The model under review builds one solid part; all positions refer to its coordinate system, in mm. A direction names the side the tool comes from. Coordinates: 2 decimals unless noted, no trailing zeros. Order: outer loops, then holes, each group sorted by start corner. A loop starts at its lowest first (then second) coordinate and runs counter-clockwise, first axis right, second up. Notation, with made-up numbers: (-13, 15.5) -> (29, 15.5) arc R17 ccw to (29, 29.5) -> close; hole circle Ø10 at (80.25, -26). An arc over 180 degrees is marked (long way). Use one line per item in the form item = value. Start each with the question number.
(1) Wall thickness on line 1 along X through (y, z) = (304.45, 5.5); line 2 along Y through (x, z) = (-935.75, 6.25); line 3 along X through (y, z) = (304.2, -3): over which ranges is each line inside the solid? List them lowest first.
(2) Take a section at C-C (x = -935). State the section outline as (y, z) points.
(3) Take a section at B-B (x = -944.25). State the section outline as (y, z) points.
(4) Take a section at D-D (y = 302.3). State the section outline as (x, z) points.
(5) Take a section at A-A (z = -7.5). State the section outline as (x, y) points.
(6) Mouldability with a two-part tool opening along X and no side actions: class faces 1 (the cylindrical face through (-942.71, 304.69, -0.13)), 2 (the cylindrical face through (-943.634, 306.887, -0.133)), 3 (the cylindrical face through (-946.211, 303.218, -0.133)), 4 (the flat face through (-934, 304, -9.5)) as +X half, -X half, draft (parallel to the pull), parting line (faces both ways), or undercut.
(7) For faces 5 (the flat face through (-930, 305.387, 0)), 6 (the flat face through (-948, 303.387, 0)), 7 (the flat face through (-930, 303.387, 0)), 8 (the flat face through (-948, 305.387, 0)), list the 3-axis set-ups (+Z, -Z, +X, -X, +Y, -Y) from which the entire face can be reached by the end or side of a thin tool; tool diameter is ignored.
(8) Insertion check: pin 1 Ø0.5 at (x, z) = (-947.5, -3.5) entering from -Y; pin 2 Ø4 at (x, z) = (-924, 6.5) entering from +Y; pin 3 Ø2 at (y, z) = (306, 0) entering from +X; pin 4 Ø1.6 at (x, y) = (-943.66, 304.39) entering from +Z. Each pin has a flat end and moves straight along its axis. Give the tip position at first contact, or say it passes through.
```python
from build123d import *

# Parameters (mm, degrees)
BOSS_EXTRUDE1_DEPTH      = 9.5
BOSS_EXTRUDE1_DEPTH_BACK = 9.5
SKETCH1_R                = 1


with BuildPart() as part:
    # Sketch1 → Boss-Extrude1 (new, two sides: drawn at the far end of the back side and taken through both)
    with BuildSketch(Plane.XY.offset(-BOSS_EXTRUDE1_DEPTH_BACK)):
        with BuildLine():
            Line((-948.662974387, 303.387338025), (-947.017076353, 303.387338025))
            ThreePointArc((-947.017076353, 303.387338025), (-946.200579773, 303.213079884), (-945.526364368, 302.720671359))
            ThreePointArc((-945.526364368, 302.720671359), (-943.662974387, 301.887338025), (-941.799584406, 302.720671359))
            ThreePointArc((-941.799584406, 302.720671359), (-941.125369002, 303.213079884), (-940.308872421, 303.387338025))
            Line((-940.308872421, 303.387338025), (-919.662974387, 303.387338025))
            ThreePointArc((-919.662974387, 303.387338025), (-919.309420997, 303.533784635), (-919.162974387, 303.887338025))
            Line((-919.162974387, 303.887338025), (-919.162974387, 304.887338025))
            ThreePointArc((-919.162974387, 304.887338025), (-919.309420997, 305.240891416), (-919.662974387, 305.387338025))
            Line((-919.662974387, 305.387338025), (-940.308872421, 305.387338025))
            ThreePointArc((-940.308872421, 305.387338025), (-941.125369002, 305.561596167), (-941.799584406, 306.054004692))
            ThreePointArc((-941.799584406, 306.054004692), (-943.662974387, 306.887338025), (-945.526364368, 306.054004692))
            ThreePointArc((-945.526364368, 306.054004692), (-946.200579773, 305.561596167), (-947.017076353, 305.387338025))
            Line((-947.017076353, 305.387338025), (-948.662974387, 305.387338025))
            ThreePointArc((-948.662974387, 305.387338025), (-949.016527778, 305.240891416), (-949.162974387, 304.887338025))
            Line((-949.162974387, 304.887338025), (-949.162974387, 303.887338025))
            ThreePointArc((-949.162974387, 303.887338025), (-949.016527778, 303.533784635), (-948.662974387, 303.387338025))
        make_face()
        with Locations((-943.662974387, 304.387338025)):
            Circle(SKETCH1_R, mode=Mode.SUBTRACT)
    extrude(amount=BOSS_EXTRUDE1_DEPTH + BOSS_EXTRUDE1_DEPTH_BACK)


solid = part.part
```
Findings:
q1.line_1 = -949.16 to -944.66, -942.66 to -919.16
q1.line_2 = 303.39 to 305.39
q1.line_3 = -949.16 to -944.65, -942.68 to -919.16
q2.outline = (303.39, -9.5) -> (305.39, -9.5) -> (305.39, 9.5) -> (303.39, 9.5) -> close
q3.outline = (301.96, -9.5) -> (303.58, -9.5) -> (303.58, 9.5) -> (301.96, 9.5) -> close; (305.2, -9.5) -> (306.82, -9.5) -> (306.82, 9.5) -> (305.2, 9.5) -> close
q4.outline = (-945.04, -9.5) -> (-942.29, -9.5) -> (-942.29, 9.5) -> (-945.04, 9.5) -> close
q5.outline = (-949.16, 303.89) arc R0.5 ccw to (-948.66, 303.39) -> (-947.02, 303.39) arc R2 cw to (-945.53, 302.72) arc R2.5 ccw to (-941.8, 302.72) arc R2 cw to (-940.31, 303.39) -> (-919.66, 303.39) arc R0.5 ccw to (-919.16, 303.89) -> (-919.16, 304.89) arc R0.5 ccw to (-919.66, 305.39) -> (-940.31, 305.39) arc R2 cw to (-941.8, 306.05) arc R2.5 ccw to (-945.53, 306.05) arc R2 cw to (-947.02, 305.39) -> (-948.66, 305.39) arc R0.5 ccw to (-949.16, 304.89) -> close; hole circle Ø2 at (-943.66, 304.39)
q6.face_1 = undercut
q6.face_2 = parting line
q6.face_3 = -X half
q6.face_4 = draft
q7.face_5 = +Z, -Z, +X, +Y
q7.face_6 = +Z, -Z, -X, -Y
q7.face_7 = +Z, -Z, +X, -Y
q7.face_8 = +Z, -Z, -X, +Y
q8.pin_1 = 303.39
q8.pin_2 = 305.39
q8.pin_3 = -919.18
q8.pin_4 = through
